Work out the finished part from the listing and answer in its coordinate system (mm). A direction names the side the tool comes from. Give positions to 0.01 mm unless a question says otherwise; leave off trailing zeros. Loops run counter-clockwise (first coordinate to the right, second up) from the corner with the lowest first, then second, coordinate; pieces in that order, holes last. Notation, with made-up numbers: (-31.5, -8) - (-8.5, -8) arc R14 cw to (-8.5, -3) - close; hole circle Ø6 at (7, -16.5). An arc over 180 degrees is marked (long way). One line per item, written item: value.
from build123d import *

# Parameters (mm, degrees)
BASE_FLANGE1_DEPTH            = 3.175
EDGE_FLANGE1_STRIP_W          = 19.05
EDGE_FLANGE1_STRIP_H          = 3.175
EDGE_FLANGE1_STRIP_CUT_DEPTH  = 37.325997284
EDGE_FLANGE1_RELIEF_W         = 20.6375
EDGE_FLANGE1_RELIEF_H         = 1.5875
EDGE_FLANGE1_RELIEF_CUT_DEPTH = 3.175
EDGE_FLANGE1_DEPTH            = 37.325997284
SKETCH15_R                    = 2.65
CUT_EXTRUDE2_DEPTH            = 10
SKETCH19_R                    = 3.15
CUT_EXTRUDE4_DEPTH            = 10


# Sheet-metal steps are written as plain solids
with BuildPart() as part:
    # Sketch3 → Base-Flange1 (new body)
    with BuildSketch(Plane(origin=(0, 0, 0), x_dir=(0, 0, -1), z_dir=(1, 0, 0))):
        with BuildLine():
            Line((83.106142408, 32.105064535), (45.780209905, 32.174606262))
            Line((45.780209905, 32.174606262), (45.780209905, 43.136168925))
            ThreePointArc((45.780209905, 43.136168925), (46.495831721, 45.713784796), (48.437851335, 47.553561406))
            Line((48.437851335, 47.553561406), (83.169236275, 65.970162941))
            Line((83.169236275, 65.970162941), (83.106142408, 32.105064535))
        make_face()
    extrude(amount=-BASE_FLANGE1_DEPTH)

    # Edge-Flange1 strip (across the edge) → Edge-Flange1 strip cut (cut)
    with BuildSketch(Plane(origin=(0, 32.174606262, -45.780209905), x_dir=(3.4914813388431334e-15, 0.999998264444559, -0.001863090945206598), z_dir=(0, -0.001863090945206598, -0.999998264444559))):
        with Locations((-3.175, -1.5875)):
            Rectangle(EDGE_FLANGE1_STRIP_W, EDGE_FLANGE1_STRIP_H)
    extrude(amount=EDGE_FLANGE1_STRIP_CUT_DEPTH, mode=Mode.SUBTRACT)

    # Edge-Flange1 relief (on the sheet) → Edge-Flange1 relief cut (cut)
    with BuildSketch(Plane(origin=(0, 38.524595242, -45.792040532), x_dir=(6.982962677686267e-15, 0.999998264444559, -0.001863090945206598), z_dir=(1, 0, 0))):
        with Locations((-8.73125, 0.79375)):
            Rectangle(EDGE_FLANGE1_RELIEF_W, EDGE_FLANGE1_RELIEF_H)
    extrude(amount=-EDGE_FLANGE1_RELIEF_CUT_DEPTH, mode=Mode.SUBTRACT)

    # Edge-Flange1 section (across the edge) → Edge-Flange1 (add)
    with BuildSketch(Plane(origin=(0, 32.174606262, -45.780209905), x_dir=(3.4914813388431334e-15, 0.999998264444559, -0.001863090945206598), z_dir=(0, -0.001863090945206598, -0.999998264444559))):
        with BuildLine():
            Line((0, 3.175), (0, 15))
            Line((0, 15), (3.175, 15))
            Line((3.175, 15), (3.175, 3.175))
            ThreePointArc((3.175, 3.175), (4.10493597, 0.92993597), (6.35, 0))
            Line((6.35, 0), (6.35, -3.175))
            ThreePointArc((6.35, -3.175), (1.859871939, -1.315128061), (0, 3.175))
        make_face()
    extrude(amount=EDGE_FLANGE1_DEPTH)

    # Sketch15 → Cut-Extrude2 (cut)
    with BuildSketch(Plane(origin=(0, 35.434781617, -0.066018335), x_dir=(1, 0, 0), z_dir=(-3.23986857388729e-15, 0.999998264444559, -0.0018630909452065992))):
        with Locations(Location((9.0875, 74.237769892, 0), (0, 0, 270))):
            Circle(SKETCH15_R)
        with Locations(Location((9.0875, 54.233380341, 0), (0, 0, 270))):
            Circle(SKETCH15_R)
    extrude(amount=-CUT_EXTRUDE2_DEPTH, mode=Mode.SUBTRACT)

    # Sketch19 → Cut-Extrude4 (cut)
    with BuildSketch(Plane.ZY.offset(3.175)):
        with Locations((-54.306440614, 43.455053514)):
            Circle(SKETCH19_R)
        with Locations((-74.30640548, 50.955053514)):
            Circle(SKETCH19_R)
    extrude(amount=-CUT_EXTRUDE4_DEPTH, mode=Mode.SUBTRACT)


solid = part.part
1. Find the intervals of material crossed by line 1 along Z through (x, y) = (-0.75, 39); line 2 along Y through (x, z) = (7.25, -47.5); line 3 along X through (y, z) = (61, -74) (3 decimals), in increasing order.
Output:
line 1: z = -83.12 to -45.79
line 2: y = 32.17 to 35.35
line 3: x = -3.175 to 0
2. Flat-ended cylindrical pins translate along their axes: pin 1 Ø5 at (y, z) = (40, -76.5) entering from +X; pin 2 Ø1 at (x, z) = (11, -63) entering from -Y; pin 3 Ø10 at (y, z) = (43.46, -54.31) entering from +X. Find the tip coordinate at first contact, or state that the pin passes through.
Output:
pin 1: stops at x = 0.15
pin 2: stops at y = 32.14
pin 3: stops at x = 0
3. Section A-A (y = 50.5) is taken. Write down the section's boundary in (x, z) (3 decimals).
Output:
outline: (-3.175, -83.14) - (0, -83.14) - (0, -77.423) - (-3.175, -77.423) - close; (-3.175, -71.189) - (0, -71.189) - (0, -53.994) - (-3.175, -53.994) - close
4. For faces 5 (the flat face through (0, 49, -69)), 6 (the flat face through (-1.565, 56.633, -65.56)), 7 (the cylindrical face through (0.955, 36.221, -64.189)), 8 (the cylindrical face through (-1.364, 34.05, -64.185)), determine the directions among +Z, -Z, +X, -X, +Y, -Y from which every point of the face is accessible in a straight line to the end or side of a thin tool.
Output:
face 5: +Z, -Z, +X, +Y
face 6: +Z, +X, -X, +Y
face 7: -Z, +X, +Y
face 8: +Z, -X, -Y
5. Section D-D (z = -53) is taken. Count the separate pieces of the cut face and the enclosed holes in it, and give its area (3 significant figures).
Output:
separate pieces: 3
enclosed holes: 0
area: 64.8 mm²
6. Section B-B (x = 10) is taken. Write down the section's boundary in (y, z).
Output:
outline: (32.11, -83.11) - (35.28, -83.11) - (35.29, -76.79) - (32.12, -76.79) - close; (32.13, -71.81) - (35.3, -71.82) - (35.33, -56.79) - (32.15, -56.78) - close; (32.16, -51.81) - (35.34, -51.81) - (35.35, -45.79) - (32.17, -45.78) - close
7. The mould has two halves that part along X. Classify faces 1 (the cylindrical face through (11.32, 33.77, -52.87)), 2 (the cylindrical face through (-1.61, 53.61, -72.61)), 3 (the flat face through (-3.175, 49, -69)), 4 (the flat face through (15, 34, -64)): released by +X, released by -X, zero draft, split by the parting line, or undercut.
Output:
face 1: undercut
face 2: zero draft
face 3: released by -X
face 4: released by +X
8. Section C-C (y = 45) is taken. Write down the section's boundary in (x, z) (3 decimals).
Output:
outline: (-3.175, -83.13) - (0, -83.13) - (0, -57.052) - (-3.175, -57.052) - close; (-3.175, -51.561) - (0, -51.561) - (0, -46.141) - (-3.175, -46.141) - close
